For this review, take the finished solid that the model builds, in its own axes (mm). A direction names the side the tool comes from. Coordinates: 2 decimals unless noted, no trailing zeros. Write each loop counter-clockwise with the first axis right and the second up, starting at its lowest first coordinate (ties: lowest second). Pieces come first, ordered by that corner, then holes.
1) Mouldability with a two-part tool opening along Y and no side actions: class faces 1 (the face through (-4.15, 16.594, 6.543)), 2 (the face through (0, 13, 15.24)), 3 (the face through (9, 9.346, 7)), 4 (the face through (9, -9.346, 7)) as pulls with the +Y half, pulls with the -Y half, needs draft (parallel to the pull), parting line crosses it, or undercut.
2) Insertion check: P1, Ø4.5, axis at y = 14.3, z = 5.08, coming from the -X side; P2, Ø2.5, axis at x = 8.5, z = 7.5, coming from the +Y side; P3, Ø1, axis at x = 9, z = 4.5, coming from the -Y side; P4, Ø2.5, axis at x = 8, y = 14.5, coming from the -Z side (3 decimals). Each pin has a flat end and moves straight along its axis. Give the tip position at first contact, or say it passes through.
3) We need section C-C on z = 9.5. Write out the cut boundary in (x, y).
4) To check wall thickness, follow line 1 along Y through (x, z) = (-1.5, 5.08); line 2 along X through (y, z) = (-12, 1.5); line 3 along Y through (x, z) = (5.25, 5.75). State the ranges of each line that lie inside material, in increasing order.
5) We need section B-B on y = 0. Write out the cut boundary in (x, z).
6) We need section D-D on x = -3.75. Write out the cut boundary in (y, z), then the cut area to 3 significant figures.
7) We need section A-A on z = 5.08. Write out the cut boundary in (x, y), then the cut area to 3 significant figures.
8) For faces 5 (the face through (-14.653, 0, 8)), 6 (the face through (0, 0, 7.874)), 7 (the face through (6.652, 14, 8)), 8 (the face through (6.652, -14, 8)), list the 3-axis set-ups (+Z, -Z, +X, -X, +Y, -Y) from which the entire face can be reached by the end or side of a thin tool; tool diameter is ignored.
from build123d import *

# Parameters (mm, degrees)
SKETCH1_W           = 29.306429484
SKETCH1_H           = 38.503943882
SKETCH1_R           = 11.303
BOSS_EXTRUDE1_DEPTH = 15.24
SKETCH4_W           = 4.826
SKETCH4_H           = 9.906
CUT_EXTRUDE1_DEPTH  = 13.335
SKETCH5_R           = 11.303
BOSS_EXTRUDE3_DEPTH = 7.874
SKETCH6_R           = 2.721770122
CUT_EXTRUDE2_DEPTH  = 31.75


with BuildPart() as part:
    # Sketch1 → Boss-Extrude1 (new body)
    with BuildSketch(Plane.XY):
        Rectangle(SKETCH1_W, SKETCH1_H)
        with Locations(Location((0, 0, 0), (0, 0, 180))):
            Circle(SKETCH1_R, mode=Mode.SUBTRACT)
    extrude(amount=BOSS_EXTRUDE1_DEPTH)

    # Sketch4 → Cut-Extrude1 (cut)
    with BuildSketch(Plane(origin=(0, 0, 0), x_dir=(-1, 0, 0), z_dir=(0, 0, -1))):
        with Locations((-9.065214742, 14.298971941)):
            Rectangle(SKETCH4_W, SKETCH4_H)
    cut_extrude1 = extrude(amount=-CUT_EXTRUDE1_DEPTH, mode=Mode.SUBTRACT)

    # Sketch5 → Boss-Extrude3 (add)
    with BuildSketch(Plane(origin=(0, 0, 0), x_dir=(-1, 0, 0), z_dir=(0, 0, -1))):
        Circle(SKETCH5_R)
    extrude(amount=-BOSS_EXTRUDE3_DEPTH)

    # Sketch6 → Cut-Extrude2 (cut)
    with BuildSketch(Plane.ZY.offset(14.653214742)):
        with Locations((5.08, 14.298971941)):
            Circle(SKETCH6_R)
    cut_extrude2 = extrude(amount=-CUT_EXTRUDE2_DEPTH, mode=Mode.SUBTRACT)

    # Mirror1: Cut-Extrude1, Cut-Extrude2 across plane
    add(cut_extrude1.mirror(Plane.ZX), mode=Mode.SUBTRACT)
    add(cut_extrude2.mirror(Plane.ZX), mode=Mode.SUBTRACT)


solid = part.part
Result:
1. face 1: undercut
1. face 2: needs draft
1. face 3: pulls with the +Y half
1. face 4: pulls with the -Y half
2. P1: passes through
2. P2: stops at y = 9.35
2. P3: stops at y = -9.35
2. P4: stops at z = 13.335
3. outline: (-14.65, -19.25) - (6.65, -19.25) - (6.65, -9.35) - (11.48, -9.35) - (11.48, -19.25) - (14.65, -19.25) - (14.65, 19.25) - (11.48, 19.25) - (11.48, 9.35) - (6.65, 9.35) - (6.65, 19.25) - (-14.65, 19.25) - close; hole circle Ø22.61 at (0, 0)
4. line 1: y = -19.25 to -17.02, -11.58 to 11.58, 17.02 to 19.25
4. line 2: x = -14.65 to 6.65, 11.48 to 14.65
4. line 3: y = -19.25 to -16.94, -11.66 to 11.66, 16.94 to 19.25
5. outline: (-14.65, 0) - (14.65, 0) - (14.65, 15.24) - (11.3, 15.24) - (11.3, 7.87) - (-11.3, 7.87) - (-11.3, 15.24) - (-14.65, 15.24) - close
6. outline: (-19.25, 0) - (19.25, 0) - (19.25, 15.24) - (10.66, 15.24) - (10.66, 7.87) - (-10.66, 7.87) - (-10.66, 15.24) - (-19.25, 15.24) - close; hole circle Ø5.44 at (-14.3, 5.08); hole circle Ø5.44 at (14.3, 5.08)
6. area: 383 mm2
7. outline: (-14.65, -19.25) - (6.65, -19.25) - (6.65, -17.02) - (-14.65, -17.02) - close; (-14.65, -11.58) - (6.65, -11.58) - (6.65, -9.35) - (11.48, -9.35) - (11.48, -11.58) - (14.65, -11.58) - (14.65, 11.58) - (11.48, 11.58) - (11.48, 9.35) - (6.65, 9.35) - (6.65, 11.58) - (-14.65, 11.58) - close; (-14.65, 17.02) - (6.65, 17.02) - (6.65, 19.25) - (-14.65, 19.25) - close; (11.48, -19.25) - (14.65, -19.25) - (14.65, -17.02) - (11.48, -17.02) - close; (11.48, 17.02) - (14.65, 17.02) - (14.65, 19.25) - (11.48, 19.25) - close
7. area: 766 mm2
8. face 5: +Z, -Z, -X, +Y, -Y
8. face 6: +Z
8. face 7: -Z, +Y
8. face 8: -Z, -Y
